from build123d import *

# Parameters (mm, degrees)
SKETCH1_W           = 58
SKETCH1_H           = 22
BOSS_EXTRUDE1_DEPTH = 1.5
SKETCH2_W           = 5
SKETCH2_H           = 5
SKETCH2_W_2         = 1.5
SKETCH2_H_2         = 4.802137959
SKETCH2_W_3         = 3
SKETCH2_H_3         = 7
SKETCH2_W_4         = 8
SKETCH2_H_4         = 8
BOSS_EXTRUDE2_DEPTH = 2.5
SKETCH3_W           = 1.5
SKETCH3_H           = 4.802137959
SKETCH3_W_2         = 5
SKETCH3_H_2         = 5
SKETCH3_W_3         = 8
SKETCH3_H_3         = 8
BOSS_EXTRUDE3_DEPTH = 3.5


with BuildPart() as part:
    # Sketch1 → Boss-Extrude1 (new body)
    with BuildSketch(Plane.XY):
        with Locations((9.718487395, 11)):
            Rectangle(SKETCH1_W, SKETCH1_H)
    extrude(amount=BOSS_EXTRUDE1_DEPTH)

    # Sketch2 → Boss-Extrude2 (add)
    with BuildSketch(Plane(origin=(0, 0, 0), x_dir=(-1, 0, 0), z_dir=(0, 0, -1))):
        with Locations((15.281512605, 18)):
            Rectangle(SKETCH2_W, SKETCH2_H)
        with Locations((18.531512605, 5.498931021)):
            Rectangle(SKETCH2_W_2, SKETCH2_H_2)
        with Locations((-37.218487395, 18)):
            Rectangle(SKETCH2_W_3, SKETCH2_H_3)
        with Locations((-33.218487395, 5.5)):
            Rectangle(SKETCH2_W_4, SKETCH2_H_4)
    extrude(amount=BOSS_EXTRUDE2_DEPTH)

    # Sketch3 → Boss-Extrude3 (add)
    with BuildSketch(Plane(origin=(0, 0, -2.5), x_dir=(-1, 0, 0), z_dir=(0, 0, -1))):
        with Locations((18.531512605, 5.498931021)):
            Rectangle(SKETCH3_W, SKETCH3_H)
        with Locations((15.281512605, 18)):
            Rectangle(SKETCH3_W_2, SKETCH3_H_2)
        with Locations((-33.218487395, 5.5)):
            Rectangle(SKETCH3_W_3, SKETCH3_H_3)
    extrude(amount=BOSS_EXTRUDE3_DEPTH)


solid = part.part
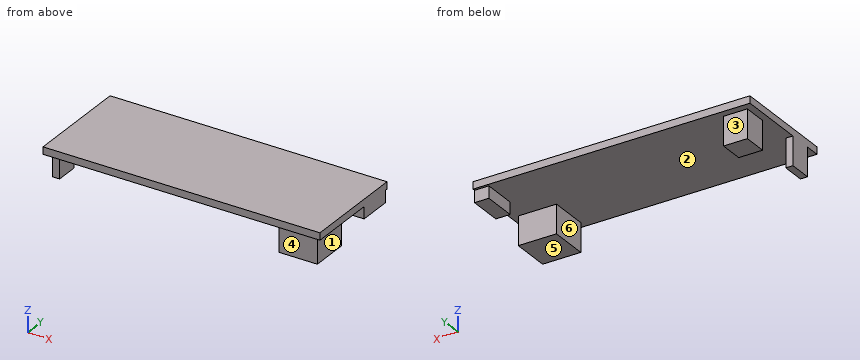
Build history of the part. All positions in model axes, mm. Face numbers are marked on the shaded views. A direction names the side the tool comes from. Give positions to 0.01 mm unless a question says otherwise; leave off trailing zeros. Order: outer loops, then holes, each group sorted by start corner. A loop starts at its lowest first (then second) coordinate and runs counter-clockwise, first axis right, second up. Notation, with made-up numbers: M 2,39.25 L 52,39.25 A31 cw 52,76.25 Z; hole C 2.25,-19 d5. An arc over 180 degrees is marked long. Use one line per item in the form item = value.
Q1. Slice it at D-D, the plane x = -2. Write the cut outline in (y, z), and give its area (3 significant figures).
Conclusion:
outline = M 0,0 L 22,0 L 22,1.5 L 0,1.5 Z
area = 33.0 mm2
Q2. Which spindle directions (+Z, -Z, +X, -X, +Y, -Y) get a long thin tool onto all of the face, cutting with end or side? Do the marked faces 4, 5 and 6. Say none if no direction does.
Conclusion:
face_4 = -Z, +X, -X, -Y
face_5 = -Z, +X, -X, +Y, -Y
face_6 = -Z, +Y, -Y
Q3. Slice it at A-A, the plane z = -3.75. Write the cut outline in (x, y).
Conclusion:
outline = M -19.28,3.1 L -17.78,3.1 L -17.78,7.9 L -19.28,7.9 Z; M -17.78,15.5 L -12.78,15.5 L -12.78,20.5 L -17.78,20.5 Z; M 29.22,1.5 L 37.22,1.5 L 37.22,9.5 L 29.22,9.5 Z
Q4. Slice it at B-B, the plane y = 18.5. Write the cut outline in (x, z), and give its area (4 significant figures).
Conclusion:
outline = M -19.28,0 L -17.78,0 L -17.78,-6 L -12.78,-6 L -12.78,0 L 35.72,0 L 35.72,-2.5 L 38.72,-2.5 L 38.72,1.5 L -19.28,1.5 Z
area = 124.5 mm2
Q5. Slice it at C-C, the plane z = -0.75. Write the cut outline in (x, y), and give its area (3 significant figures).
Conclusion:
outline = M -19.28,3.1 L -17.78,3.1 L -17.78,7.9 L -19.28,7.9 Z; M -17.78,15.5 L -12.78,15.5 L -12.78,20.5 L -17.78,20.5 Z; M 29.22,1.5 L 37.22,1.5 L 37.22,9.5 L 29.22,9.5 Z; M 35.72,14.5 L 38.72,14.5 L 38.72,21.5 L 35.72,21.5 Z
area = 117 mm2
Q6. Pin check, flat tips, straight feed: P1, Ø1.5, axis at y = 17, z = -3, coming from the -X side; P2, Ø1.2, axis at x = 37, z = -1, coming from the +Y side; P3, Ø2.5, axis at x = 38, y = 19.5, coming from the -Z side. Stop position of each tip, or through.
Conclusion:
P1 = -17.78
P2 = 21.5
P3 = -2.5
Q7. Wall check: probe 1 along X at (y, z) = (6.25, -2.5); probe 2 along Z at (x, y) = (9, 7.75); probe 3 along X at (y, z) = (8.5, -0.5). Give the ranges that are in metal, low to high.
Conclusion:
probe_1 = -19.28 to -17.78, 29.22 to 37.22
probe_2 = 0 to 1.5
probe_3 = 29.22 to 37.22
Q8. Pull direction X, two halves, no side cores. Call the marked faces 1, 2 and 3: released by +X, released by -X, zero draft, split by the parting line, or undercut.
Conclusion:
face_1 = released by +X
face_2 = undercut
face_3 = zero draft
